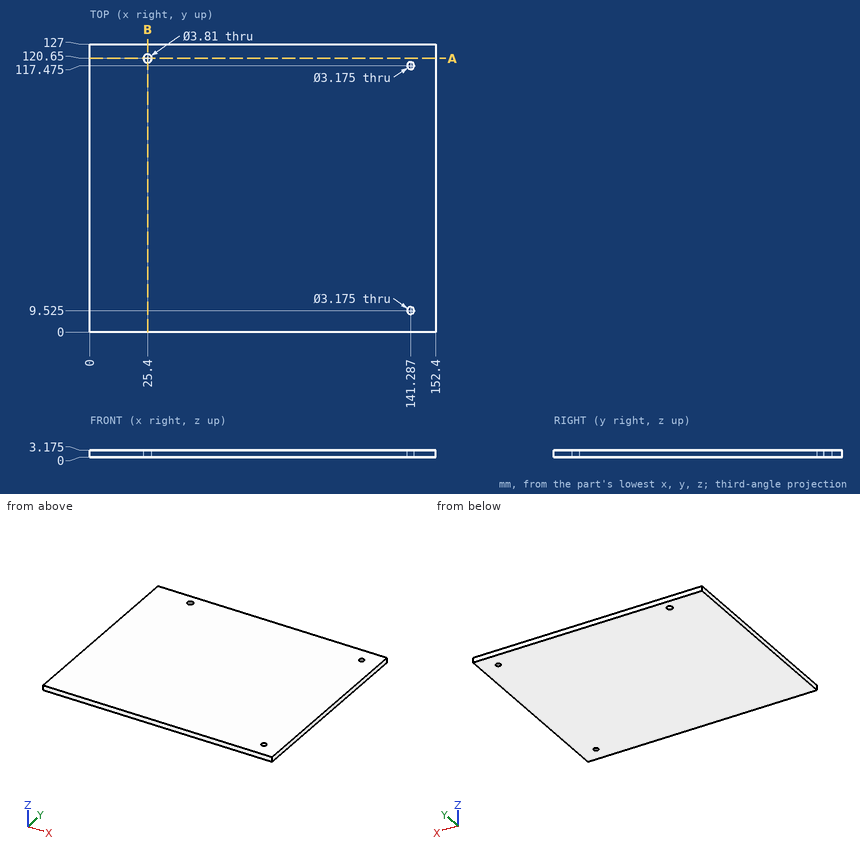
Verification items for this drawing (mm, ordinates from the low corner). Give positions to 0.01 mm unless a question says otherwise; leave off trailing zeros. Loops run counter-clockwise (first coordinate to the right, second up) from the corner with the lowest first, then second, coordinate; pieces in that order, holes last. Notation, with made-up numbers: (67, 38.25) - (79, 38.25) arc R13 cw to (79, 62.25) - close; hole circle Ø4 at (72, -10). An arc over 180 degrees is marked (long way). Write item = value, one per line. Start each with the question number.
Q1. Cross-section at B-B, the plane x = 25.4. Enter the section's corners in (y, z) (1 decimal), and give its area (3 significant figures).
Q2. Thickness scan on line 1 (X direction, y = 120.65, z = 1.6) (1 decimal); line 2 (Y direction, x = 25.4, z = 1.6) (1 decimal); line 3 (Y direction, x = 142, z = 2.2) (1 decimal). Record the ranges inside material, lowest first.
Q3. Cross-section at A-A, the plane y = 120.65. Enter the section's corners in (x, z) (1 decimal).
Q4. Depth check by flat-ended pin: P1, Ø1.9, axis at x = 141.29, y = 117.48, coming from the -Z side. Enter the tip coordinate at first touch or a pass-through.
Answer key:
q1.outline = (0, 0) - (118.7, 0) - (118.7, 3.2) - (0, 3.2) - close; (122.6, 0) - (127, 0) - (127, 3.2) - (122.6, 3.2) - close
q1.area = 391 mm^2
q2.line_1 = 0 to 23.5, 27.3 to 152.4
q2.line_2 = 0 to 118.7, 122.6 to 127
q2.line_3 = 0 to 8.1, 10.9 to 116.1, 118.9 to 127
q3.outline = (0, 0) - (23.5, 0) - (23.5, 3.2) - (0, 3.2) - close; (27.3, 0) - (152.4, 0) - (152.4, 3.2) - (27.3, 3.2) - close
q4.P1 = through
